```python
from build123d import *

# Parameters (mm, degrees)
SKETCH1_R                                      = 11.1125
SKETCH1_R_2                                    = 3.175
SKETCH1_R_3                                    = 3.96875
SKETCH1_R_4                                    = 4
BOSS_EXTRUDE1_DEPTH                            = 3.175
CSK_FOR_6_FLAT_HEAD_MACHINE_SCREW1_D           = 3.6576
CSK_FOR_6_FLAT_HEAD_MACHINE_SCREW1_DEPTH       = 8
CSK_FOR_6_FLAT_HEAD_MACHINE_SCREW1_CSINK_D     = 7.0866
CSK_FOR_6_FLAT_HEAD_MACHINE_SCREW1_CSINK_ANGLE = 82
CSK_FOR_6_FLAT_HEAD_MACHINE_SCREW1_TIP         = 1.0988539


with BuildPart() as part:
    # Sketch1 → Boss-Extrude1 (new body)
    with BuildSketch(Plane.XY):
        Polygon((-23.359070214, 22.5), (131.2, 22.5), (131.2, -85.2), (12.315929786, -85.2), (12.315929786, -50.95), (-20.184070214, -50.95), (-20.184070214, -35.2), (-23.359070214, -35.2), align=None)
        Circle(SKETCH1_R, mode=Mode.SUBTRACT)
        with Locations((112.2, -41.275)):
            Circle(SKETCH1_R, mode=Mode.SUBTRACT)
        with Locations((-13.834070214, -43.2)):
            Circle(SKETCH1_R_2, mode=Mode.SUBTRACT)
        with Locations((45, -40)):
            Circle(SKETCH1_R_2, mode=Mode.SUBTRACT)
        with Locations((63.404393546, -6.8)):
            Circle(SKETCH1_R_2, mode=Mode.SUBTRACT)
        with Locations((88.602925496, -30.405847557)):
            Circle(SKETCH1_R_3, mode=Mode.SUBTRACT)
        with Locations((112.2, -15.295)):
            Circle(SKETCH1_R_3, mode=Mode.SUBTRACT)
        with Locations((87.828697203, -50.275)):
            Circle(SKETCH1_R_3, mode=Mode.SUBTRACT)
        with Locations((101.330847557, -64.872074504)):
            Circle(SKETCH1_R_3, mode=Mode.SUBTRACT)
        with Locations((121.2, -65.646302797)):
            Circle(SKETCH1_R_3, mode=Mode.SUBTRACT)
        with Locations((84.102828318, 12.5)):
            Circle(SKETCH1_R_4, mode=Mode.SUBTRACT)
    extrude(amount=-BOSS_EXTRUDE1_DEPTH)

    # CSK for #6 Flat Head Machine Screw1
    with Locations(Plane(origin=(0, 0, -3.175), x_dir=(-1, 0, 0), z_dir=(0, 0, -1))):
        with Locations((-125.136432586, -35.922550846), (-106.847550846, -28.338567414), (-99.263567414, -46.627449154), (-117.552449154, -54.211432586), (-5.352449154, -12.936432586), (-12.936432586, 5.352449154), (5.352449154, 12.936432586), (12.936432586, -5.352449154)):
            CounterSinkHole(CSK_FOR_6_FLAT_HEAD_MACHINE_SCREW1_D / 2, CSK_FOR_6_FLAT_HEAD_MACHINE_SCREW1_CSINK_D / 2, depth=CSK_FOR_6_FLAT_HEAD_MACHINE_SCREW1_DEPTH, counter_sink_angle=CSK_FOR_6_FLAT_HEAD_MACHINE_SCREW1_CSINK_ANGLE)
            with Locations((0, 0, -(CSK_FOR_6_FLAT_HEAD_MACHINE_SCREW1_DEPTH + CSK_FOR_6_FLAT_HEAD_MACHINE_SCREW1_TIP / 2))):  # 118° drill point
                Cone(0, CSK_FOR_6_FLAT_HEAD_MACHINE_SCREW1_D / 2, CSK_FOR_6_FLAT_HEAD_MACHINE_SCREW1_TIP, mode=Mode.SUBTRACT)


solid = part.part
```
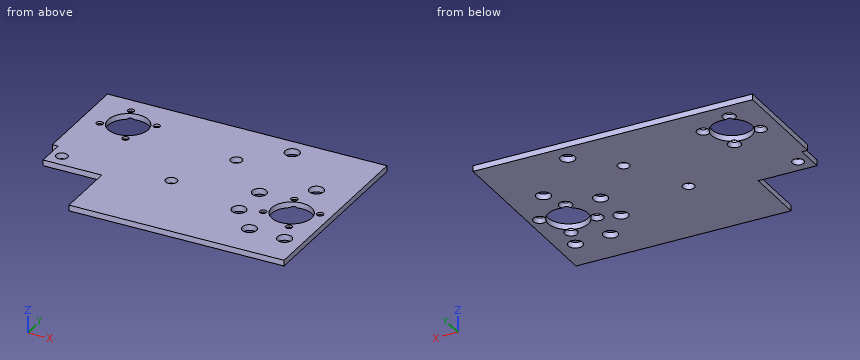
Here's how the part is built. I have some questions about the finished solid (model axes, mm). Round coordinates to 2 decimals unless told otherwise and drop trailing zeros. Order: outer loops, then holes, each group sorted by start corner. A loop starts at its lowest first (then second) coordinate and runs counter-clockwise, first axis right, second up. Notation, with made-up numbers: M 38.25,50 L 83.25,50 A29 ccw 83.25,89 Z; hole C 7,34.25 d1. An arc over 180 degrees is marked long. Answer in a Markdown table with one row per item.
Item 1: Imagine slicing it at A-A, the plane x = 112.2. Write out the boundary of the cut face in (y, z) (1 decimal), and give its area (3 significant figures).
A:
| item | result |
|---|---|
| outline | M -85.2,-3.2 L -52.4,-3.2 L -52.4,0 L -85.2,0 Z; M -30.2,-3.2 L -19.3,-3.2 L -19.3,0 L -30.2,0 Z; M -11.3,-3.2 L 22.5,-3.2 L 22.5,0 L -11.3,0 Z |
| area | 246 mm2 |
Item 2: I'm going to push flat-ended pins straight in: pin 1 (6.5 mm diameter, centred on x = 121.2, y = -65.65, fed in from +Z); pin 2 (5 mm diameter, centred on x = 99.26, y = -46.63, fed in from -Z); pin 3 (1 mm diameter, centred on y = -43, z = -1.5, fed in from -X); pin 4 (4 mm diameter, centred on x = 106.85, y = -28.34, fed in from -Z). Where does each tip first touch, or does it pass through?
A:
| item | result |
|---|---|
| pin 1 | passes through |
| pin 2 | stops at z = -1.98 |
| pin 3 | stops at x = -20.18 |
| pin 4 | stops at z = -1.4 |
Item 3: If I drill on L1, parallel to X at y = -66.5, z = -1.25; L2, parallel to X at y = -36, z = -2.4 (3 decimals); L3, parallel to X at y = -41, z = -0.4, over which ranges is the centre line in solid material (lowest first)? Write a range as from..to.
A:
| item | result |
|---|---|
| L1 | x = 12.32..97.71, 104.95..117.32, 125.08..131.2 |
| L2 | x = -20.184..102.419, 121.981..122.268, 128.005..131.2 |
| L3 | x = -20.18..-16.12, -11.54..41.99, 48.01..101.09, 123.31..131.2 |
Item 4: Imagine slicing it at C-C, the plane y = 0. Write out the boundary of the cut face in (x, z) (1 decimal).
A:
| item | result |
|---|---|
| outline | M -23.4,-3.2 L -11.1,-3.2 L -11.1,0 L -23.4,0 Z; M 11.1,-3.2 L 131.2,-3.2 L 131.2,0 L 11.1,0 Z |
Item 5: Imagine slicing it at B-B, the plane x = 45. Write out the boundary of the cut face in (y, z) (3 decimals).
A:
| item | result |
|---|---|
| outline | M -85.2,-3.175 L -43.175,-3.175 L -43.175,0 L -85.2,0 Z; M -36.825,-3.175 L 22.5,-3.175 L 22.5,0 L -36.825,0 Z |
